Check sheet for the modelled part. Datum: model origin and axes. Units: mm. Give positions to 0.01 mm unless a question says otherwise; leave off trailing zeros. Write each loop counter-clockwise with the first axis right and the second up, starting at its lowest first coordinate (ties: lowest second). Pieces come first, ordered by that corner, then holes. Notation, with made-up numbers: (26.5, 7.5) -> (58.5, 7.5) arc R16 ccw to (58.5, 23.5) -> close; hole circle Ø5 at (28.25, -3). An arc over 180 degrees is marked (long way). Use a Markdown table: item, result. Add a question column.
1. Cross-section at A-A (x = 0). Enter the section's corners in (y, z), then the cut area to 3 significant figures.
2. Gauge pin test, flat ends, axial feed: P1, Ø1.5, axis at y = 80.5, z = -9.5, coming from the +X side; P2, Ø6, axis at x = -7, y = 171, coming from the -Z side; P3, Ø5, axis at y = 165, z = -8, coming from the +X side (3 decimals). Record the tip position at first contact, or that the pin passes through.
3. Scan lines: probe 1 along X at (y, z) = (153, 0); probe 2 along Z at (x, y) = (-0.25, 78.5); probe 3 along Z at (x, y) = (-3.75, 104). Record each from-to range of solid material in increasing order. Write a range as [from, to].
4. Cross-section at B-B (z = 0). Enter the section's corners in (x, y).
5. Release check for a two-part mould opening along Z. For faces 1 (the cylindrical face through (3.755, 111.537, 11.923)), 2 (the cylindrical face through (-4.034, 111.532, -0.896)), 3 (the flat face through (-5, 226.231, 0)) record: released by +Z, released by -Z, zero draft, split by the parting line, or undercut.
6. Cross-section at C-C (y = 163.5). Enter the section's corners in (x, z), then the cut area to 3 significant figures.
from build123d import *

# Parameters (mm, degrees)
SKETCH1_R           = 12.5
BOSS_EXTRUDE1_DEPTH = 226.231428
SKETCH2_R           = 4.132090217
CUT_EXTRUDE1_DEPTH  = 227.921041367
CHAMFER1_SIZE       = 0.291606
CHAMFER1_SIZE_2     = 0.289934


with BuildPart() as part:
    # Sketch1 → Boss-Extrude1 (new body)
    with BuildSketch(Plane(origin=(0, 0, 0), x_dir=(1, 0, 0), z_dir=(0, 1, 0))):
        with Locations(Location((0, 0, 0), (0, 0, 270))):
            Circle(SKETCH1_R)
    extrude(amount=BOSS_EXTRUDE1_DEPTH)

    # Sketch2 → Cut-Extrude1 (cut, through all)
    with BuildSketch(Plane(origin=(0, 0, 0), x_dir=(1, 0, 0), z_dir=(0, 1, 0))):
        with Locations(Location((0, 0, 0), (0, 0, 270))):
            Circle(SKETCH2_R)
    extrude(amount=CUT_EXTRUDE1_DEPTH, mode=Mode.SUBTRACT)

    # Chamfer1
    # the kernel refuses this chamfer: 0.291606, 0.289934 mm, written as the material it takes off along each edge
    with BuildSketch(Plane(origin=(0, 0, 0), x_dir=(0, 0, 1), z_dir=(-1, 0, 0))) as chamfer1_piece_1:
        Polygon((12.5, CHAMFER1_SIZE), (12.5 - CHAMFER1_SIZE_2, 0), (12.5, 0), align=None)
    revolve(axis=Axis((0, 0, 0), (0, 1, 0)), mode=Mode.SUBTRACT)
    with BuildSketch(Plane(origin=(0, 226.231428, 0), x_dir=(0, 0, 1), z_dir=(-1, 0, 0))) as chamfer1_piece_2:
        Polygon((12.5, -CHAMFER1_SIZE_2), (12.5 - CHAMFER1_SIZE, 0), (12.5, 0), align=None)
    revolve(axis=Axis((0, 226.231428, 0), (0, 1, 0)), mode=Mode.SUBTRACT)


solid = part.part
Worked answers:
| question | item | result |
|---|---|---|
| 1 | outline | (0, -12.21) -> (0.29, -12.5) -> (225.94, -12.5) -> (226.23, -12.21) -> (226.23, -4.13) -> (0, -4.13) -> close; (0, 4.13) -> (226.23, 4.13) -> (226.23, 12.21) -> (225.94, 12.5) -> (0.29, 12.5) -> (0, 12.21) -> close |
| 1 | area | 3,790 mm² |
| 2 | P1 | stops at x = 8.93 |
| 2 | P2 | stops at z = -11.84 |
| 2 | P3 | stops at x = 11.225 |
| 3 | probe 1 | x = [-12.5, -4.13], [4.13, 12.5] |
| 3 | probe 2 | z = [-12.5, -4.12], [4.12, 12.5] |
| 3 | probe 3 | z = [-11.92, -1.74], [1.74, 11.92] |
| 4 | outline | (-12.5, 0.29) -> (-12.21, 0) -> (-4.13, 0) -> (-4.13, 226.23) -> (-12.21, 226.23) -> (-12.5, 225.94) -> close; (4.13, 0) -> (12.21, 0) -> (12.5, 0.29) -> (12.5, 225.94) -> (12.21, 226.23) -> (4.13, 226.23) -> close |
| 5 | face 1 | split by the parting line |
| 5 | face 2 | undercut |
| 5 | face 3 | zero draft |
| 6 | outline | circle Ø25 at (0, 0); hole circle Ø8.26 at (0, 0) |
| 6 | area | 437 mm² |
